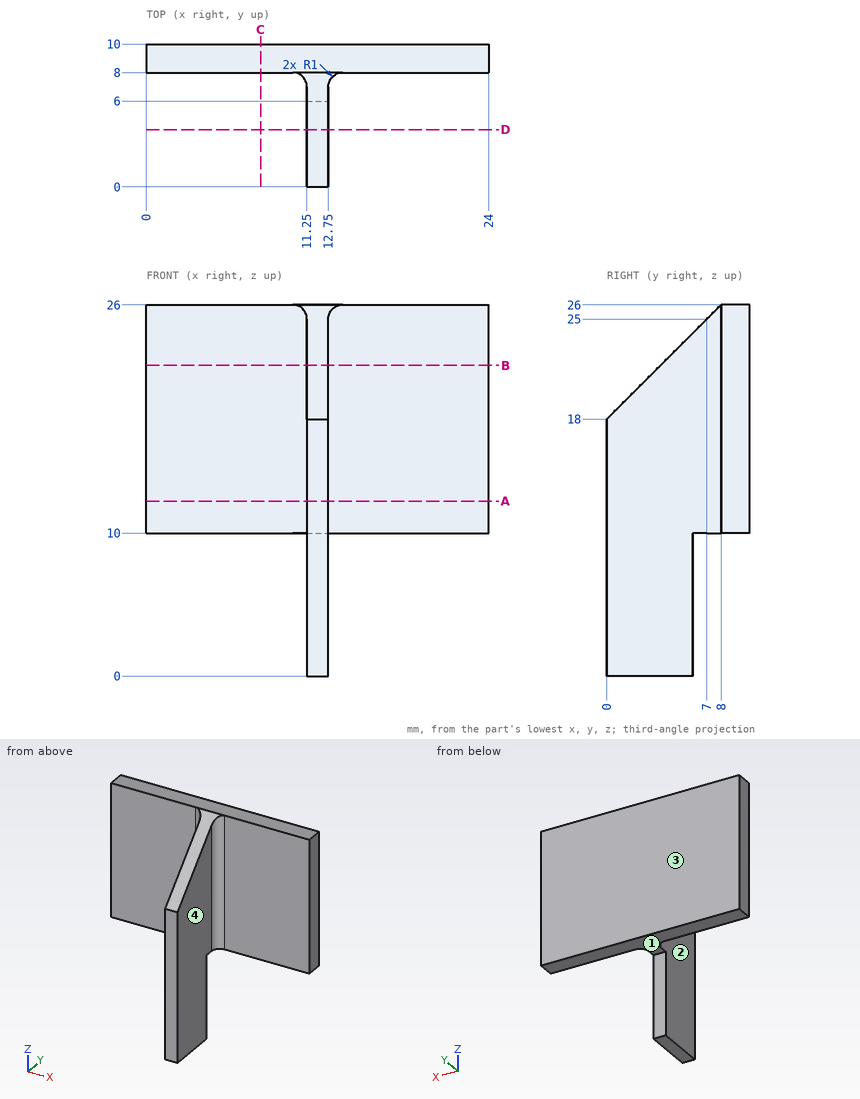
Verification items for this drawing (mm, ordinates from the low corner). A direction names the side the tool comes from. Give positions to 0.01 mm unless a question says otherwise; leave off trailing zeros. Loops run counter-clockwise (first coordinate to the right, second up) from the corner with the lowest first, then second, coordinate; pieces in that order, holes last. Notation, with made-up numbers: M -21,62.25 L -6,62.25 A19 cw -6,97.25 Z; hole C 44,77 d4. An arc over 180 degrees is marked long. Answer as a JSON object with one key per item and string values. Group by question number.
Item 1: Sectioned sample at D-D on y = 4. Record the boundary of the cut face in (x, z).
Item 2: Access from +Z, -Z, +X, -X, +Y, -Y to the whole of each face (thin tool, end or side, straight path). Record for the marked faces 1, 2, 3 and 4.
Item 3: Material ranges on L1, parallel to Y at x = 23.25, z = 24; L2, parallel to X at y = 1.5, z = 10.5; L3, parallel to X at y = 7.5, z = 14.25, recorded low to high.
Item 4: Gauge pin test, flat ends, axial feed: pin 1 (5 mm diameter, centred on x = 19.5, z = 17.5, fed in from -Y); pin 2 (2 mm diameter, centred on y = 6, z = 16.5, fed in from -X); pin 3 (3.5 mm diameter, centred on y = 3.5, z = 15, fed in from +X). Record the tip position at first contact, or that the pin passes through.
Item 5: Sectioned sample at B-B on z = 21.75. Record the boundary of the cut face in (x, y), plus the area to 3 significant figures.
Item 6: Sectioned sample at A-A on z = 12.25. Record the boundary of the cut face in (x, y), plus the area to 3 significant figures.
Item 7: Sectioned sample at C-C on x = 8. Record the boundary of the cut face in (y, z).
Findings below:
{
 "1": {"outline": "M 11.25,0 L 12.75,0 L 12.75,22 L 11.25,22 Z"},
 "2": {"face 1": "-Z, +X, -X, +Y", "face 2": "+Z, -Z, -X, -Y", "face 3": "+Z, -Z, +X, -X, +Y", "face 4": "+Z, -Z, +X, -Y"},
 "3": {"L1": "8 to 10", "L2": "11.25 to 12.75", "L3": "11.12 to 12.88"},
 "4": {"pin 1": "y = 8", "pin 2": "x = 11.25", "pin 3": "x = 12.75"},
 "5": {"outline": "M 0,8 L 10.25,8 A1 cw 11.25,7 L 11.25,3.75 L 12.75,3.75 L 12.75,7 A1 cw 13.75,8 L 24,8 L 24,10 L 0,10 Z", "area": "54.8 mm2"},
 "6": {"outline": "M 0,8 L 10.25,8 A1 cw 11.25,7 L 11.25,0 L 12.75,0 L 12.75,7 A1 cw 13.75,8 L 24,8 L 24,10 L 0,10 Z", "area": "60.4 mm2"},
 "7": {"outline": "M 8,10 L 10,10 L 10,26 L 8,26 Z"}
}
